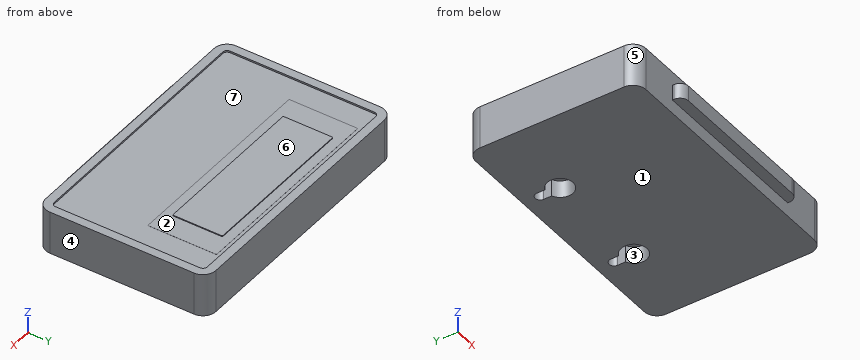
from build123d import *

# Parameters (mm, degrees)
F0_W      = 80.01
F0_H      = 50.292
F1_DEPTH  = 6.35
F2_R      = 3.81
F4_DEPTH  = 0.508
F5_W      = 49.53
F5_H      = 4.572
F6_DEPTH  = 3.048
F7_R      = 2.54
F9_DEPTH  = 0.0254
F11_DEPTH = 0.254
F13_DEPTH = 5.08


with BuildPart() as f1:
    # F0 (on Top) → F1 (new body, symmetric)
    with BuildSketch(Plane.XY):
        Rectangle(F0_W, F0_H)
    extrude(amount=F1_DEPTH, both=True)

    # F2
    f2_edges = [f1.edges().sort_by_distance(p)[0] for p in [
        (-40.005, -25.146, 0),
        (40.005, -25.146, 0),
        (40.005, 25.146, 0),
        (-40.005, 25.146, 0),
    ]]
    fillet(f2_edges, radius=F2_R)

    # F3 (on face) → F4 (cut)
    with BuildSketch(Plane.XY.offset(6.35)):
        with BuildLine():
            ThreePointArc((37.474391, 21.336), (37.099666, 22.240666), (36.195, 22.615391))
            Line((36.195, 22.615391), (-36.195, 22.615391))
            ThreePointArc((-36.195, 22.615391), (-37.099666, 22.240666), (-37.474391, 21.336))
            Line((-37.474391, 21.336), (-37.474391, -21.336))
            ThreePointArc((-37.474391, -21.336), (-37.099666, -22.240666), (-36.195, -22.615391))
            Line((-36.195, -22.615391), (36.195, -22.615391))
            ThreePointArc((36.195, -22.615391), (37.099666, -22.240666), (37.474391, -21.336))
            Line((37.474391, -21.336), (37.474391, 21.336))
        make_face()
    extrude(amount=-F4_DEPTH, mode=Mode.SUBTRACT)

    # F5 (on face) → F6 (join)
    with BuildSketch(Plane.XZ.offset(25.146)):
        Rectangle(F5_W, F5_H)
    extrude(amount=F6_DEPTH)

    # F7
    f7_edges = [f1.edges().sort_by_distance(p)[0] for p in [
        (24.765, -28.194, 0),
        (-24.765, -28.194, 0),
    ]]
    fillet(f7_edges, radius=F7_R)

    # F8 (on face) → F9 (join)
    with BuildSketch(Plane.XY.offset(5.842)):
        with BuildLine():
            Line((30.099, 21.336), (-30.099, 21.336))
            ThreePointArc((-30.099, 21.336), (-30.278605, 21.261605), (-30.353, 21.082))
            Line((-30.353, 21.082), (-30.353, 1.27))
            ThreePointArc((-30.353, 1.27), (-30.278605, 1.090395), (-30.099, 1.016))
            Line((-30.099, 1.016), (30.099, 1.016))
            ThreePointArc((30.099, 1.016), (30.278605, 1.090395), (30.353, 1.27))
            Line((30.353, 1.27), (30.353, 21.082))
            ThreePointArc((30.353, 21.082), (30.278605, 21.261605), (30.099, 21.336))
        make_face()
    extrude(amount=F9_DEPTH)

    # F10 (on face) → F11 (join)
    with BuildSketch(Plane.XY.offset(5.8674)):
        with BuildLine():
            Line((23.495, 18.542), (-23.495, 18.542))
            ThreePointArc((-23.495, 18.542), (-23.674605, 18.467605), (-23.749, 18.288))
            Line((-23.749, 18.288), (-23.749, 4.064))
            ThreePointArc((-23.749, 4.064), (-23.674605, 3.884395), (-23.495, 3.81))
            Line((-23.495, 3.81), (23.495, 3.81))
            ThreePointArc((23.495, 3.81), (23.674605, 3.884395), (23.749, 4.064))
            Line((23.749, 4.064), (23.749, 18.288))
            ThreePointArc((23.749, 18.288), (23.674605, 18.467605), (23.495, 18.542))
        make_face()
    extrude(amount=F11_DEPTH)

    # F12 (on face) → F13 (cut)
    with BuildSketch(Plane(origin=(0, 0, -6.35), x_dir=(1, 0, 0), z_dir=(0, 0, -1))):
        with BuildLine():
            Line((14.401857, -17.68688), (14.401857, -20.053012))
            ThreePointArc((14.401857, -20.053012), (14.4018, -20.066), (14.401857, -20.078988))
            ThreePointArc((14.401857, -20.078988), (15.881494, -21.539186), (17.3482, -20.066))
            Line((17.3482, -20.066), (17.3482, -17.686856))
            ThreePointArc((17.3482, -17.686856), (15.874969, -10.3632), (14.401857, -17.68688))
        make_face()
        with BuildLine():
            ThreePointArc((-14.401857, -17.68688), (-15.874969, -10.3632), (-17.3482, -17.686856))
            Line((-17.3482, -17.686856), (-17.3482, -20.066))
            ThreePointArc((-17.3482, -20.066), (-15.881494, -21.539186), (-14.401857, -20.078988))
            ThreePointArc((-14.401857, -20.078988), (-14.4018, -20.066), (-14.401857, -20.053012))
            Line((-14.401857, -20.053012), (-14.401857, -17.68688))
        make_face()
    extrude(amount=-F13_DEPTH, mode=Mode.SUBTRACT)


solid = f1.part
For this review, take the finished solid that the model builds, in its own axes (mm). Face numbers are marked on the shaded views. A direction names the side the tool comes from. Give positions to 0.01 mm unless a question says otherwise; leave off trailing zeros. Order: outer loops, then holes, each group sorted by start corner. A loop starts at its lowest first (then second) coordinate and runs counter-clockwise, first axis right, second up. Notation, with made-up numbers: M 74,64.25 L 109,64.25 A23 cw 109,87.25 Z; hole C -6.75,87 d9. An arc over 180 degrees is marked long. Answer in a Markdown table with one row per item. Add a question column.
(1) Mouldability with a two-part tool opening along Y and no side actions: class the marked faces 4, 5, 6 and 7 as +Y half, -Y half, draft (parallel to the pull), parting line (faces both ways), or undercut.
(2) For pin 1 (5 mm diameter, centred on x = -24.5, z = 4, fed in from -Y); pin 2 (7.5 mm diameter, centred on x = 1, y = 12, fed in from +Z); pin 3 (3.5 mm diameter, centred on x = -6, y = -27, fed in from -Z), all flat-tipped, find the tip position at first contact; note any pin that passes through.
(3) Consider section D-D on z = -0.25. State the section outline as (x, y) points (3 decimals).
(4) Consider section B-B on z = -4. Give the number of separate pieces and of enclosed holes in the cut face, and give its area (3 significant figures).
(5) For the marked faces 1, 2 and 3, list the 3-axis set-ups (+Z, -Z, +X, -X, +Y, -Y) from which the entire face can be reached by the end or side of a thin tool; tool diameter is ignored.
(6) Consider section C-C on y = 5.5. State the section outline as (x, z) points (3 decimals), and give its area (3 significant figures).
(7) Wall thickness on probe 1 along Y at (x, z) = (35.5, -2.75); probe 2 along Z at (x, y) = (21.5, 22.5); probe 3 along Z at (x, y) = (-26.5, 16.5): over which ranges is each line inside the solid? List them lowest first. Write a range as [from, to].
Evaluation:
| question | item | result |
|---|---|---|
| 1 | face 4 | draft |
| 1 | face 5 | -Y half |
| 1 | face 6 | undercut |
| 1 | face 7 | undercut |
| 2 | pin 1 | stops at y = -28.15 |
| 2 | pin 2 | stops at z = 6.12 |
| 2 | pin 3 | stops at z = -2.29 |
| 3 | outline | M -40.005,-21.336 A3.81 ccw -36.195,-25.146 L -24.765,-25.146 L -24.765,-25.654 A2.54 ccw -22.225,-28.194 L 22.225,-28.194 A2.54 ccw 24.765,-25.654 L 24.765,-25.146 L 36.195,-25.146 A3.81 ccw 40.005,-21.336 L 40.005,21.336 A3.81 ccw 36.195,25.146 L -36.195,25.146 A3.81 ccw -40.005,21.336 Z |
| 4 | separate pieces | 1 |
| 4 | enclosed holes | 2 |
| 4 | area | 3,900 mm^2 |
| 5 | face 1 | -Z, +X, -X, +Y, -Y |
| 5 | face 2 | +Z |
| 5 | face 3 | -Z |
| 6 | outline | M -40.005,-6.35 L 40.005,-6.35 L 40.005,6.35 L 37.474,6.35 L 37.474,5.842 L 30.353,5.842 L 30.353,5.867 L 23.749,5.867 L 23.749,6.121 L -23.749,6.121 L -23.749,5.867 L -30.353,5.867 L -30.353,5.842 L -37.474,5.842 L -37.474,6.35 L -40.005,6.35 Z |
| 6 | area | 992 mm^2 |
| 7 | probe 1 | y = [-25.15, 25.15] |
| 7 | probe 2 | z = [-6.35, 5.84] |
| 7 | probe 3 | z = [-6.35, 5.87] |
